from build123d import *

# Parameters (mm, degrees)
F0_R     = 14.2875
F1_DEPTH = 35
F2_DEPTH = 50.8


with BuildPart() as f1:
    # F0 (on Front) → F1 (new body)
    with BuildSketch(Plane.XZ):
        with BuildLine():
            Line((11.8201890877, 26.0156444266), (3.2047751505, 28.3947185447))
            ThreePointArc((3.2047751505, 28.3947185447), (-28.5220001461, -1.739578301), (6.631814894, -27.7947774989))
            Line((6.631814894, -27.7947774989), (9.0167764908, -27.1150948129))
            ThreePointArc((9.0167764908, -27.1150948129), (23.1752563441, -16.7164026748), (28.575, 0))
            ThreePointArc((28.575, 0), (24.0238686329, 15.47205096), (11.8201890877, 26.0156444266))
        make_face()
        with BuildLine():
            ThreePointArc((-13.4703841816, 4.7625), (0, 14.2875), (13.4703841816, 4.7625))
            Line((13.4703841816, 4.7625), (19.05, 4.7625))
            Line((19.05, 4.7625), (19.05, -4.7625))
            Line((19.05, -4.7625), (13.4703841816, -4.7625))
            ThreePointArc((13.4703841816, -4.7625), (0, -14.2875), (-13.4703841816, -4.7625))
            Line((-13.4703841816, -4.7625), (-19.05, -4.7625))
            Line((-19.05, -4.7625), (-19.05, 4.7625))
            Line((-19.05, 4.7625), (-13.4703841816, 4.7625))
        make_face(mode=Mode.SUBTRACT)
        with BuildLine():
            Line((45.0618756476, 16.8362321877), (11.8201890877, 26.0156444266))
            ThreePointArc((11.8201890877, 26.0156444266), (24.0238686329, 15.47205096), (28.575, 0))
            ThreePointArc((28.575, 0), (23.1752563441, -16.7164026748), (9.0167764908, -27.1150948129))
            Line((9.0167764908, -27.1150948129), (45.0698397536, -16.8404459854))
            ThreePointArc((45.0698397536, -16.8404459854), (34.9250005327, -0.0045050825), (45.0618756476, 16.8362321877))
        make_face()
        with BuildLine():
            ThreePointArc((73.025, 0), (63.8011762931, 16.3201948351), (45.0618756476, 16.8362321877))
            ThreePointArc((45.0618756476, 16.8362321877), (34.9250005327, -0.0045050825), (45.0698397536, -16.8404459854))
            ThreePointArc((45.0698397536, -16.8404459854), (63.8050355367, -16.3178706131), (73.025, 0))
        make_face()
        with Locations((53.975, 0)):
            Circle(F0_R, mode=Mode.SUBTRACT)
    extrude(amount=F1_DEPTH)

    # F0 (on Front) → F2 (join)
    with BuildSketch(Plane.XZ):
        with BuildLine():
            Line((11.8201890877, 26.0156444266), (3.2047751505, 28.3947185447))
            ThreePointArc((3.2047751505, 28.3947185447), (-28.5220001461, -1.739578301), (6.631814894, -27.7947774989))
            Line((6.631814894, -27.7947774989), (9.0167764908, -27.1150948129))
            ThreePointArc((9.0167764908, -27.1150948129), (23.1752563441, -16.7164026748), (28.575, 0))
            ThreePointArc((28.575, 0), (24.0238686329, 15.47205096), (11.8201890877, 26.0156444266))
        make_face()
        with BuildLine():
            ThreePointArc((-13.4703841816, 4.7625), (0, 14.2875), (13.4703841816, 4.7625))
            Line((13.4703841816, 4.7625), (19.05, 4.7625))
            Line((19.05, 4.7625), (19.05, -4.7625))
            Line((19.05, -4.7625), (13.4703841816, -4.7625))
            ThreePointArc((13.4703841816, -4.7625), (0, -14.2875), (-13.4703841816, -4.7625))
            Line((-13.4703841816, -4.7625), (-19.05, -4.7625))
            Line((-19.05, -4.7625), (-19.05, 4.7625))
            Line((-19.05, 4.7625), (-13.4703841816, 4.7625))
        make_face(mode=Mode.SUBTRACT)
    extrude(amount=F2_DEPTH)


solid = f1.part
CAD build for the part. Positions are in the model's coordinates, mm. A direction names the side the tool comes from. Give positions to 0.01 mm unless a question says otherwise; leave off trailing zeros. Write each loop counter-clockwise with the first axis right and the second up, starting at its lowest first coordinate (ties: lowest second). Pieces come first, ordered by that corner, then holes. Notation, with made-up numbers: M -17,-21 L 5,-21 A35 cw 5,13 Z; hole C -2.75,-11.75 d3. An arc over 180 degrees is marked long. Put each result on its own line as item: value. Start each with the question number.
(1) Mould opens along Z. For faces 1 (the face through (22, 0, 0)), 2 (the face through (-28.556, -25.044, -1.043)), 3 (the face through (-16, -25, -4.762)) say: +Z half, -Z half, draft (parallel to the pull), parting line (faces both ways), or undercut.
(2) Which spindle directions (+Z, -Z, +X, -X, +Y, -Y) get a long thin tool onto all of the face, cutting with end or side? Do faces 4 (the face through (-13, -50.8, 7)), 5 (the face through (0.246, -25.044, -14.285)). Say none if no direction does.
(3) Probe L1, parallel to Z at x = 49, y = -18; L2, parallel to Z at x = 16.5, y = -37; L3, parallel to X at y = -46, z = -3.5. List the from-to ranges inside material, lowest first.
(4) Band-saw the part on C-C, the plane z = -1.5. Write the cut outline in (x, y).
(5) Band-saw the part on A-A, the plane x = 0. Write the cut outline in (y, z) (1 decimal).
(6) Band-saw the part on B-B, the plane y = -23. Give the number of separate pieces and of enclosed holes in the cut face, and give its area (3 significant figures).
(7) Band-saw the part on D-D, the plane x = 65. Write the cut outline in (y, z).
(8) Flat gauge pins, fed straight in: pin 1 Ø3 at (x, y) = (15.5, -30) entering from +Z; pin 2 Ø10 at (x, y) = (60, -28.5) entering from -Z; pin 3 Ø16 at (x, z) = (53.5, -9) entering from -Y. Where does each tip first touch, or does it go through?
Response values:
1. face 1: draft
1. face 2: parting line
1. face 3: undercut
2. face 4: +Z, -Z, +X, -X, -Y
2. face 5: +Y, -Y
3. L1: z = -18.39 to -13.39, 13.39 to 18.39
3. L2: z = -23.33 to -4.76, 4.76 to 23.33
3. L3: x = -28.36 to -19.05, 19.05 to 28.36
4. outline: M -28.54,-50.8 L -19.05,-50.8 L -19.05,0 L -28.54,0 Z; M 19.05,-50.8 L 28.54,-50.8 L 28.54,-35 L 39.77,-35 L 39.77,0 L 19.05,0 Z; M 68.18,-35 L 72.97,-35 L 72.97,0 L 68.18,0 Z
5. outline: M -50.8,-28.6 L 0,-28.6 L 0,-14.3 L -50.8,-14.3 Z; M -50.8,14.3 L 0,14.3 L 0,28.6 L -50.8,28.6 Z
6. separate pieces: 1
6. enclosed holes: 2
6. area: 2,880 mm2
7. outline: M -35,-15.54 L 0,-15.54 L 0,-9.09 L -35,-9.09 Z; M -35,9.09 L 0,9.09 L 0,15.54 L -35,15.54 Z
8. pin 1: stops at z = 25.41
8. pin 2: stops at z = -19.02
8. pin 3: stops at y = -35
